Work out the finished part from the listing and answer in its coordinate system (mm). Face numbers are marked on the shaded views. Round coordinates to 2 decimals unless told otherwise and drop trailing zeros. Write each loop counter-clockwise with the first axis right and the second up, starting at its lowest first coordinate (ties: lowest second). Pieces come first, ordered by that corner, then holes.
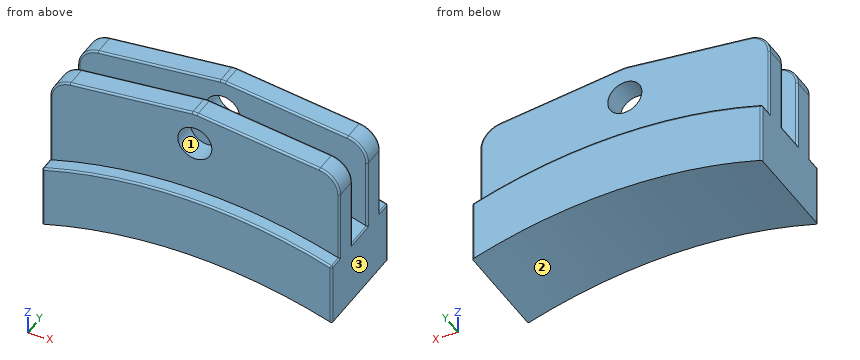
from build123d import *

# Parameters (mm, degrees)
F1_DEPTH = 28.575
F0_R     = 9.525
F2_DEPTH = 20.6375
F3_DEPTH = 7.9375
F7_R     = 1.016


with BuildPart() as f1:
    # F0 (on Front) → F1 (new body, symmetric)
    with BuildSketch(Plane.XZ):
        with BuildLine():
            ThreePointArc((-80.9625, 0), (0, 12.4151634214), (80.9625, 0))
            Line((80.9625, 0), (80.9625, 34.925))
            ThreePointArc((80.9625, 34.925), (0, 47.3401634214), (-80.9625, 34.925))
            Line((-80.9625, 34.925), (-80.9625, 0))
        make_face()
    extrude(amount=F1_DEPTH, both=True)

    # F0 (on Front) → F2 (join, symmetric)
    with BuildSketch(Plane.XZ):
        with BuildLine():
            ThreePointArc((-80.9625, 34.925), (0, 47.3401634214), (80.9625, 34.925))
            Line((80.9625, 34.925), (80.9625, 74.4315304023))
            ThreePointArc((80.9625, 74.4315304023), (77.7528984326, 82.8708631715), (69.7463838441, 87.0445430772))
            Line((69.7463838441, 87.0445430772), (1.4838838441, 95.0754254301))
            ThreePointArc((1.4838838441, 95.0754254301), (0, 95.1624127552), (-1.4838838441, 95.0754254301))
            Line((-1.4838838441, 95.0754254301), (-69.7463838441, 87.0445430772))
            ThreePointArc((-69.7463838441, 87.0445430772), (-77.7528984326, 82.8708631715), (-80.9625, 74.4315304023))
            Line((-80.9625, 74.4315304023), (-80.9625, 34.925))
        make_face()
        with Locations((0, 76.2)):
            Circle(F0_R, mode=Mode.SUBTRACT)
    extrude(amount=F2_DEPTH, both=True)

    # F0 (on Front) → F3 (cut, symmetric)
    with BuildSketch(Plane.XZ):
        with BuildLine():
            ThreePointArc((-80.9625, 34.925), (0, 47.3401634214), (80.9625, 34.925))
            Line((80.9625, 34.925), (80.9625, 74.4315304023))
            ThreePointArc((80.9625, 74.4315304023), (77.7528984326, 82.8708631715), (69.7463838441, 87.0445430772))
            Line((69.7463838441, 87.0445430772), (1.4838838441, 95.0754254301))
            ThreePointArc((1.4838838441, 95.0754254301), (0, 95.1624127552), (-1.4838838441, 95.0754254301))
            Line((-1.4838838441, 95.0754254301), (-69.7463838441, 87.0445430772))
            ThreePointArc((-69.7463838441, 87.0445430772), (-77.7528984326, 82.8708631715), (-80.9625, 74.4315304023))
            Line((-80.9625, 74.4315304023), (-80.9625, 34.925))
        make_face()
        with Locations((0, 76.2)):
            Circle(F0_R, mode=Mode.SUBTRACT)
    extrude(amount=F3_DEPTH, both=True, mode=Mode.SUBTRACT)

    # F7
    f7_edges = [f1.edges().sort_by_distance(p)[0] for p in [
        (80.9625, 24.60625, 34.925),
        (80.9625, -24.60625, 34.925),
        (-80.9625, 24.60625, 34.925),
        (-80.9625, -24.60625, 34.925),
        (-80.9625, 0, 34.925),
        (80.9625, 0, 34.925),
        (80.9625, 28.575, 17.4625),
        (80.9625, -28.575, 17.4625),
        (-80.9625, 28.575, 17.4625),
        (-80.9625, -28.575, 17.4625),
        (0, -28.575, 47.340163),
        (0, 28.575, 47.340163),
        (-80.9625, -20.6375, 54.678265),
        (-80.9625, -7.9375, 54.678265),
        (80.9625, 20.6375, 54.678265),
        (80.9625, 7.9375, 54.678265),
    ]]
    fillet(f7_edges, radius=F7_R)


solid = f1.part
Q1. Find section C-C (z = 76.2). Count the separate pieces of the cut face and the enclosed holes in it, plus the area to 3 significant figures.
Q2. Find the intervals of material crossed by L1, parallel to Y at x = -18, z = 81.5; L2, parallel to X at y = 19, z = 82; L3, parallel to Z at x = -70.5, y = 16, in increasing order.
Q3. Given pin 1 (6 mm diameter, centred on x = 38.5, z = 49.5, fed in from -Y); pin 2 (6 mm diameter, centred on x = -49, y = 18.5, fed in from +Z); pin 3 (1.5 mm diameter, centred on x = -31, y = 11, fed in from +Z), each flat-ended and moving along its own axis, determine where each tip first touches the part or whether it passes through.
Q4. Find section B-B (y = -0.5). Determine the outline of the cut face in (x, z), plus the area to 3 significant figures.
Q5. The mould has two halves that part along Z. Classify the marked faces 1, 2 and 3: +Z half, -Z half, draft (parallel to the pull), parting line (faces both ways), or undercut.
Report:
1. separate pieces: 4
1. enclosed holes: 0
1. area: 3,620 mm2
2. L1: y = -20.64 to -7.94, 7.94 to 20.64
2. L2: x = -78.46 to -7.56, 7.56 to 78.46
2. L3: z = 3.06 to 86.93
3. pin 1: stops at y = -20.64
3. pin 2: stops at z = 89.84
3. pin 3: stops at z = 91.69
4. outline: (-80.96, 0) arc R270.2 cw to (80.96, 0) - (80.96, 34.18) arc R1.02 ccw to (80.25, 35.15) arc R270.2 ccw to (-80.25, 35.15) arc R1.02 ccw to (-80.96, 34.18) - close
4. area: 5,660 mm2
5. face 1: undercut
5. face 2: -Z half
5. face 3: draft
